Can you work these out from the model? Positions are in its coordinate system, mm. Face numbers are marked on the shaded views. A direction names the side the tool comes from. Give positions to 0.01 mm unless a question says otherwise; leave off trailing zeros. Order: outer loops, then holes, each group sorted by start corner. A loop starts at its lowest first (then second) coordinate and runs counter-clockwise, first axis right, second up. Notation, with made-up numbers: (89, -13.5) - (101, -13.5) arc R12 cw to (101, -9.5) - close; hole circle Ø1 at (-4.5, 32.25). An arc over 180 degrees is marked (long way). One line per question, with ' | ' between items.
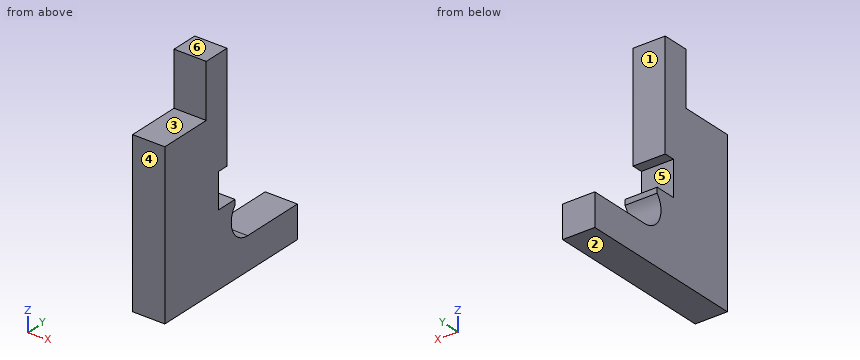
```python
from build123d import *

# Parameters (mm, degrees)
BOSS_EXTRUDE1_DEPTH = 6


with BuildPart() as part:
    # Sketch1 → Boss-Extrude1 (new body)
    with BuildSketch(Plane(origin=(0, 0, 0), x_dir=(0, 0, -1), z_dir=(1, 0, 0))):
        with BuildLine():
            Line((3.96875, 0), (3.96875, 12))
            Line((3.96875, 12), (10, 12))
            Line((10, 12), (10, -20))
            Line((10, -20), (-20, -20))
            Line((-20, -20), (-20, -10))
            Line((-20, -10), (-30, -10))
            Line((-30, -10), (-30, -5))
            Line((-30, -5), (-10.03125, -5))
            Line((-10.03125, -5), (-10.03125, -7))
            Line((-10.03125, -7), (-3.53125, -7))
            Line((-3.53125, -7), (-3.53125, -3.056754815))
            Line((-3.53125, -3.056754815), (-2.53125, -3.056754815))
            ThreePointArc((-2.53125, -3.056754815), (1.68894614, -3.591439475), (3.96875, 0))
        make_face()
    extrude(amount=BOSS_EXTRUDE1_DEPTH)


solid = part.part
```
(1) If I drill on line 1 (Z direction, x = 2.95, y = -6); line 2 (Y direction, x = 2.2, z = 27); line 3 (Z direction, x = 1.35, y = -18), over which ranges is the centre line in solid material (lowest first)?
Answer below:
line 1: -10 to 3.53, 10.03 to 30 | line 2: -10 to -5 | line 3: -10 to 20
(2) Will these pins go through, and if not, where does the flat tip stop? pin 1 (3 mm diameter, centred on x = 4, y = -14, fed in from +Z); pin 2 (3 mm diameter, centred on x = 4.5, z = 20, fed in from +Y); pin 3 (3 mm diameter, centred on x = 1.5, y = 5.5, fed in from +Z); pin 4 (1.5 mm diameter, centred on y = 5, z = -3.5, fed in from +X).
Answer below:
pin 1: z = 20 | pin 2: y = -5 | pin 3: z = -3.97 | pin 4: x = 6
(3) On a 3-axis mill with a long thin cutter (end or side, diameter ignored), from which of +Z, -Z, +X, -X, +Y, -Y can I reach the whole of each face in a straight line? I mean the marked faces 1, 2 and 3. Say none if no direction works.
Answer below:
face 1: +Z, +X, -X, +Y | face 2: -Z, +X, -X, +Y, -Y | face 3: +Z, +X, -X, -Y
(4) Imagine slicing it at D-D (y = -15). List the corners of the cut face in (x, z) for me, and give its area (3 significant figures).
Answer below:
outline: (0, -10) - (6, -10) - (6, 20) - (0, 20) - close | area: 180 mm^2
(5) Imagine slicing it at C-C (z = 5). List the corners of the cut face in (x, y) for me.
Answer below:
outline: (0, -20) - (6, -20) - (6, -7) - (0, -7) - close
(6) Imagine slicing it at B-B (x = 3.3). List the corners of the cut face in (y, z) for me, and give its area (3 significant figures).
Answer below:
outline: (-20, -10) - (12, -10) - (12, -3.97) - (0, -3.97) arc R3.97 cw to (-3.06, 2.53) - (-3.06, 3.53) - (-7, 3.53) - (-7, 10.03) - (-5, 10.03) - (-5, 30) - (-10, 30) - (-10, 20) - (-20, 20) - close | area: 602 mm^2
(7) If we mould it in two halves opening along Z, with no side actions, what happens to the marked faces 4, 5 and 6? For each: released by +Z, released by -Z, zero draft, split by the parting line, or undercut.
Answer below:
face 4: zero draft | face 5: undercut | face 6: released by +Z
(8) Imagine slicing it at A-A (y = -5.5). List the corners of the cut face in (x, z) for me.
Answer below:
outline: (0, -10) - (6, -10) - (6, 3.53) - (0, 3.53) - close; (0, 10.03) - (6, 10.03) - (6, 30) - (0, 30) - close
